```python
from build123d import *

# Parameters (mm, degrees)
BOSS_EXTRUDE1_DEPTH           = 12
FILLET2_R                     = 5
CSK_FOR_M3_SFHCS1_D           = 3.2
CSK_FOR_M3_SFHCS1_DEPTH       = 20
CSK_FOR_M3_SFHCS1_CSINK_D     = 6.72
CSK_FOR_M3_SFHCS1_CSINK_ANGLE = 90
CSK_FOR_M3_SFHCS1_TIP         = 0.96137699
SKETCH2_R                     = 9
BOSS_EXTRUDE2_DEPTH           = 18
SKETCH5_R                     = 17.5
BOSS_EXTRUDE3_DEPTH           = 12
FILLET3_R                     = 10


with BuildPart() as part:
    # Sketch1 → Boss-Extrude1 (new body)
    with BuildSketch(Plane.XY):
        Polygon((-7, 10), (-19, 10), (-19, 0), (0, 0), (0, 49), (-7, 49), align=None)
    extrude(amount=BOSS_EXTRUDE1_DEPTH)

    # Fillet2
    fillet2_edges = [part.edges().sort_by_distance(p)[0] for p in [
        (-7, 10, 6),
        (0, 0, 6),
    ]]
    fillet(fillet2_edges, radius=FILLET2_R)

    # CSK for M3 SFHCS1
    with Locations(Plane(origin=(0, 0, 0), x_dir=(0, 0, -1), z_dir=(1, 0, 0))):
        with Locations((-6, 5)):
            CounterSinkHole(CSK_FOR_M3_SFHCS1_D / 2, CSK_FOR_M3_SFHCS1_CSINK_D / 2, depth=CSK_FOR_M3_SFHCS1_DEPTH, counter_sink_angle=CSK_FOR_M3_SFHCS1_CSINK_ANGLE)
            with Locations((0, 0, -(CSK_FOR_M3_SFHCS1_DEPTH + CSK_FOR_M3_SFHCS1_TIP / 2))):  # 118° drill point
                Cone(0, CSK_FOR_M3_SFHCS1_D / 2, CSK_FOR_M3_SFHCS1_TIP, mode=Mode.SUBTRACT)

    # Sketch2 → Boss-Extrude2 (add)
    with BuildSketch(Plane.ZY.offset(7)):
        with Locations(Location((6, 49, 0), (0, 0, 228.189685104))):
            Circle(SKETCH2_R)
    extrude(amount=BOSS_EXTRUDE2_DEPTH)

    # Sketch5 → Boss-Extrude3 (add)
    with BuildSketch(Plane(origin=(-7, 0, 0), x_dir=(0, 0, -1), z_dir=(1, 0, 0))):
        with Locations(Location((-6, 49, 0), (0, 0, 90))):
            Circle(SKETCH5_R)
    extrude(amount=-BOSS_EXTRUDE3_DEPTH)

    # Fillet3
    # the kernel refuses this fillet: 10 mm, written as the material it adds along each edge
    with BuildSketch(Plane(origin=(-7, 8.712237742, 0), x_dir=(0, 0, -1), z_dir=(0, 1, 0))) as fillet3_piece_1_section:
        with BuildLine():
            CenterArc((9.539392014, -10), FILLET3_R, 90, 72.542396876)
            Line((0, -7), (0, 0))
            Line((0, 0), (9.539392014, 0))
        make_face()
    fillet3_piece_1 = extrude(amount=40.287762258, mode=Mode.PRIVATE)
    fillet3_piece_1 = fillet3_piece_1 & Plane(origin=(-7, 49, 6), x_dir=(0, 1, 0), z_dir=(1, 0, 0)) * Cylinder(17.5, 119, mode=Mode.PRIVATE)
    add(fillet3_piece_1)
    with BuildSketch(Plane(origin=(-7, 49, 0), x_dir=(0, 1, 0), z_dir=(0, 0, 1))) as fillet3_piece_2:
        with BuildLine():
            CenterArc((9.539392014, -10), FILLET3_R, 90, 72.542396876)
            Line((0, -7), (0, 0))
            Line((0, 0), (9.539392014, 0))
        make_face()
    extrude(amount=12)
    with BuildSketch(Plane(origin=(-7, 49, 12), x_dir=(1, 0, 0), z_dir=(0, -1, 0))) as fillet3_piece_3_section:
        with BuildLine():
            CenterArc((10, 9.539392014), FILLET3_R, 180, 72.542396876)
            Line((0, 9.539392014), (0, 0))
            Line((0, 0), (7, 0))
        make_face()
    fillet3_piece_3 = extrude(amount=40.287762258, mode=Mode.PRIVATE)
    fillet3_piece_3 = fillet3_piece_3 & Plane(origin=(-7, 49, 6), x_dir=(0, 1, 0), z_dir=(1, 0, 0)) * Cylinder(17.5, 119, mode=Mode.PRIVATE)
    add(fillet3_piece_3)
    with BuildSketch(Plane(origin=(-7, 8.712237742, 0), x_dir=(0, 0, -1), z_dir=(0, 1, 0))) as fillet3_piece_4a_section:
        with BuildLine():
            CenterArc((9.539392014, -10), FILLET3_R, 90, 72.542396876)
            Line((0, -7), (0, 0))
            Line((0, 0), (9.539392014, 0))
        make_face()
    fillet3_piece_4a = extrude(amount=64.136242294, mode=Mode.PRIVATE)
    fillet3_piece_4a = fillet3_piece_4a & Plane(origin=(-7, 49, 6), x_dir=(0, 1, 0), z_dir=(1, 0, 0)) * Cylinder(17.5, 167, mode=Mode.PRIVATE)
    fillet3_piece_4a = split(fillet3_piece_4a, bisect_by=Plane(origin=(-7, 49, 0), z_dir=(0, 1, 0)), keep=Keep.TOP, mode=Mode.PRIVATE)
    with BuildSketch(Plane(origin=(-7, 49, -23.848480035), x_dir=(0, 1, 0), z_dir=(0, 0, 1))) as fillet3_piece_4b_section:
        with BuildLine():
            CenterArc((9.539392014, -10), FILLET3_R, 90, 72.542396876)
            Line((0, -7), (0, 0))
            Line((0, 0), (9.539392014, 0))
        make_face()
    fillet3_piece_4b = extrude(amount=35.848480035, mode=Mode.PRIVATE)
    fillet3_piece_4b = fillet3_piece_4b & Plane(origin=(-7, 49, 6), x_dir=(0, 1, 0), z_dir=(1, 0, 0)) * Cylinder(17.5, 110, mode=Mode.PRIVATE)
    fillet3_piece_4b = split(fillet3_piece_4b, bisect_by=Plane(origin=(-7, 49, 0), z_dir=(0, 0, -1)), keep=Keep.TOP, mode=Mode.PRIVATE)
    fillet3_piece_4 = fillet3_piece_4a & fillet3_piece_4b
    add(fillet3_piece_4)
    with BuildSketch(Plane(origin=(-7, 72.848480035, 12), x_dir=(1, 0, 0), z_dir=(0, -1, 0))) as fillet3_piece_5a_section:
        with BuildLine():
            CenterArc((10, 9.539392014), FILLET3_R, 180, 72.542396876)
            Line((0, 9.539392014), (0, 0))
            Line((0, 0), (7, 0))
        make_face()
    fillet3_piece_5a = extrude(amount=64.136242294, mode=Mode.PRIVATE)
    fillet3_piece_5a = fillet3_piece_5a & Plane(origin=(-7, 49, 6), x_dir=(0, 1, 0), z_dir=(1, 0, 0)) * Cylinder(17.5, 167, mode=Mode.PRIVATE)
    fillet3_piece_5a = split(fillet3_piece_5a, bisect_by=Plane(origin=(-7, 49, 12), z_dir=(0, 1, 0)), keep=Keep.TOP, mode=Mode.PRIVATE)
    with BuildSketch(Plane(origin=(-7, 49, 0), x_dir=(0, 1, 0), z_dir=(0, 0, 1))) as fillet3_piece_5b_section:
        with BuildLine():
            CenterArc((9.539392014, -10), FILLET3_R, 90, 72.542396876)
            Line((0, -7), (0, 0))
            Line((0, 0), (9.539392014, 0))
        make_face()
    fillet3_piece_5b = extrude(amount=35.848480035, mode=Mode.PRIVATE)
    fillet3_piece_5b = split(fillet3_piece_5b, bisect_by=Plane(origin=(-7, 49, 12), z_dir=(0, 0, 1)), keep=Keep.TOP, mode=Mode.PRIVATE)
    fillet3_piece_5b = fillet3_piece_5b & Plane(origin=(-7, 49, 6), x_dir=(0, 1, 0), z_dir=(1, 0, 0)) * Cylinder(17.5, 110, mode=Mode.PRIVATE)
    fillet3_piece_5 = fillet3_piece_5a & fillet3_piece_5b
    add(fillet3_piece_5)


solid = part.part
```
The model under review builds one solid part; all positions refer to its coordinate system, in mm. A direction names the side the tool comes from. Coordinates: 2 decimals unless noted, no trailing zeros. Order: outer loops, then holes, each group sorted by start corner. A loop starts at its lowest first (then second) coordinate and runs counter-clockwise, first axis right, second up. Notation, with made-up numbers: (40.5, 55.5) -> (98.5, 55.5) arc R13 ccw to (98.5, 59.5) -> close; hole circle Ø7 at (36, 65.25). An arc over 180 degrees is marked (long way). Answer in a Markdown table with one row per item. Add a question column.
Item 1: Machinability: for faces 1 (the flat face through (-19, 57, -2)), 2 (the flat face through (-7, 49, 22)), 3 (the flat face through (-5, 13, 0)), 4 (the flat face through (-19, 6.2, 4.6)), which of the approach directions +Z, -Z, +X, -X, +Y, -Y give a long, thin tool a straight path to every point of the face, cutting with its end or side? Answer none if there is none.
Item 2: We need section A-A on x = -13.5. Write out the cut boundary in (y, z).
Item 3: We need section B-B on z = 6. Write out the cut boundary in (x, y), plus the area to 3 significant figures.
Item 4: Clearance check with flat-ended pins moving along their axes: pin 1 (4 mm diameter, centred on y = 63, z = 1.5, fed in from +X); pin 2 (9.5 mm diameter, centred on y = 27.5, z = 6.5, fed in from -X); pin 3 (5.5 mm diameter, centred on x = -6.5, y = 17.5, fed in from -Z). State where each tip first meets the part, or that it passes through.
Item 5: We need section C-C on z = 10.5. Write out the cut boundary in (x, y), plus the area to 3 significant figures.
Item 6: Mouldability with a two-part tool opening along Z and no side actions: class faces 5 (the conical face through (-1.479, 6.865, 5.755)), 6 (the cylindrical face through (-5.11, 45.1, -3.69)), 7 (the cylindrical face through (-10.5, 3.58, 6.74)), 8 (the flat face through (0, 27, 6)) as +Z half, -Z half, draft (parallel to the pull), parting line (faces both ways), or undercut.
Item 7: We need section D-D on y = 27.5. Write out the cut boundary in (x, z), plus the area to 3 significant figures.
Item 8: To check wall thickness, follow probe 1 along Z at (x, y) = (-11.75, 5); probe 2 along X at (y, z) = (38.5, 2); probe 3 along Y at (x, z) = (-5.5, 6). State the ranges of each line that lie inside material, in increasing order.
Final values:
| question | item | result |
|---|---|---|
| 1 | face 1 | -X |
| 1 | face 2 | +Z, +X, +Y, -Y |
| 1 | face 3 | -Z, +X, -X, -Y |
| 1 | face 4 | +Z, -Z, -X, -Y |
| 2 | outline | (0, 0) -> (10, 0) -> (10, 12) -> (0, 12) -> close; circle Ø35 at (49, 6); hole circle Ø3.2 at (5, 6) |
| 3 | outline | (-25, 40) -> (-19, 40) -> (-19, 31.5) -> (-7, 31.5) -> (-7, 15) arc R5 cw to (-12, 10) -> (-19, 10) -> (-19, 6.6) -> (-1.76, 6.6) -> (0, 8.36) -> (0, 49) arc R10 cw to (-7, 58.54) -> (-7, 66.5) -> (-19, 66.5) -> (-19, 58) -> (-25, 58) -> close; (-19, 0) -> (-5, 0) arc R5 ccw to (-0.74, 2.38) -> (-1.76, 3.4) -> (-19, 3.4) -> close |
| 3 | area | 946 mm2 |
| 4 | pin 1 | stops at x = -7 |
| 4 | pin 2 | stops at x = -19 |
| 4 | pin 3 | stops at z = 0 |
| 5 | outline | (-25, 41.21) -> (-19, 41.21) -> (-19, 32.09) -> (-7, 32.09) -> (-7, 15) arc R5 cw to (-12, 10) -> (-19, 10) -> (-19, 0) -> (-5, 0) arc R5 ccw to (0, 5) -> (0, 49) arc R10 cw to (-7, 58.54) -> (-7, 65.91) -> (-19, 65.91) -> (-19, 56.79) -> (-25, 56.79) -> close |
| 5 | area | 980 mm2 |
| 6 | face 5 | undercut |
| 6 | face 6 | -Z half |
| 6 | face 7 | undercut |
| 6 | face 8 | draft |
| 7 | outline | (-7, 0) -> (0, 0) -> (0, 12) -> (-7, 12) -> close |
| 7 | area | 84.0 mm2 |
| 8 | probe 1 | z = 0 to 4.4, 7.6 to 12 |
| 8 | probe 2 | x = -19 to 0 |
| 8 | probe 3 | y = 0 to 3.4, 6.6 to 53.27 |
